```python
from build123d import *

# Parameters (mm, degrees)
SKETCH1_R           = 9
BOSS_EXTRUDE1_DEPTH = 66
SKETCH2_R           = 8.5
BOSS_EXTRUDE2_DEPTH = 2
SKETCH3_R           = 8
CUT_EXTRUDE1_DEPTH  = 1.5
SKETCH4_R           = 3
BOSS_EXTRUDE3_DEPTH = 1
FILLET1_R           = 1
CHAMFER1_SIZE       = 2


with BuildPart() as part:
    # Sketch1 → Boss-Extrude1 (new body)
    with BuildSketch(Plane.XY):
        Circle(SKETCH1_R)
    extrude(amount=BOSS_EXTRUDE1_DEPTH)

    # Sketch2 → Boss-Extrude2 (add)
    with BuildSketch(Plane(origin=(0, 0, 0), x_dir=(-1, 0, 0), z_dir=(0, 0, -1))):
        Circle(SKETCH2_R)
    extrude(amount=BOSS_EXTRUDE2_DEPTH)

    # Sketch3 → Cut-Extrude1 (cut)
    with BuildSketch(Plane(origin=(0, 0, -2), x_dir=(-1, 0, 0), z_dir=(0, 0, -1))):
        Circle(SKETCH3_R)
    extrude(amount=-CUT_EXTRUDE1_DEPTH, mode=Mode.SUBTRACT)

    # Sketch4 → Boss-Extrude3 (add)
    with BuildSketch(Plane(origin=(0, 0, -0.5), x_dir=(-1, 0, 0), z_dir=(0, 0, -1))):
        with Locations((0, 4)):
            Circle(SKETCH4_R)
        with Locations((0, -4)):
            Circle(SKETCH4_R)
    extrude(amount=BOSS_EXTRUDE3_DEPTH)

    # Fillet1
    fillet1_edges = [part.edges().sort_by_distance(p)[0] for p in [
        (3, 4, -1.5),
        (3, -4, -1.5),
    ]]
    fillet(fillet1_edges, radius=FILLET1_R - 0.0001)  # a hair under: the kernel refuses the full size

    # Chamfer1
    chamfer1_edges = [part.edges().sort_by_distance(p)[0] for p in [
        (-9, 0, 66),
    ]]
    chamfer(chamfer1_edges, length=CHAMFER1_SIZE)


solid = part.part
```
Design review of the part built by this model. Coordinates are the model's own, in mm. A direction names the side the tool comes from. Coordinates: 2 decimals unless noted, no trailing zeros. Loops run counter-clockwise (first coordinate to the right, second up) from the corner with the lowest first, then second, coordinate; pieces in that order, holes last. Notation, with made-up numbers: M 55,49 L 88,49 A13 cw 88,74 Z; hole C 76,-11.5 d1. An arc over 180 degrees is marked long. One line per question, with ' | ' between items.
(1) Wall thickness on probe 1 along Y at (x, z) = (0, -1.1); probe 2 along Y at (x, z) = (0, -1.2); probe 3 along Z at (x, y) = (2.5, 1.5): over which ranges is each line inside the solid? List them lowest first.
Filled in:
probe 1: y = -8.5 to -8, -6.8 to -1.2, 1.2 to 6.8, 8 to 8.5 | probe 2: y = -8.5 to -8, -6.71 to -1.29, 1.29 to 6.71, 8 to 8.5 | probe 3: z = -0.5 to 66
(2) Draft analysis for pull direction Y (two halves, no side actions). For faces 3 (the face through (-1.172, 8.923, 31.552)), 4 (the face through (0, -4, -1.5)), 5 (the face through (8, -3.3, 0)), state which applies: released by +Y, released by -Y, zero draft, split by the parting line, or undercut.
Filled in:
face 3: split by the parting line | face 4: undercut | face 5: zero draft
(3) We need section C-C (z = 37.5). Give the boundary of the cut face in (x, y), and give its area (3 significant figures).
Filled in:
outline: C 0,0 d18 | area: 254 mm^2
(4) For pin 1 Ø5 at (y, z) = (5.5, 37.5) entering from +X; pin 2 Ø8 at (x, y) = (-3, -1) entering from -Z; pin 3 Ø5 at (x, z) = (-7, 27) entering from +Y; pin 4 Ø8 at (y, z) = (-2.5, 39) entering from -X, all flat-tipped, find the tip position at first contact; note any pin that passes through.
Filled in:
pin 1: stops at x = 8.49 | pin 2: stops at z = -1.5 | pin 3: stops at y = 7.79 | pin 4: stops at x = -9
(5) Machinability: for faces 1 (the face through (0, 0, 66)), 2 (the face through (-4.57, 7.167, -0.986)), which of the approach directions +Z, -Z, +X, -X, +Y, -Y give a long, thin tool a straight path to every point of the face, cutting with its end or side? Answer none if there is none.
Filled in:
face 1: +Z, +X, -X, +Y, -Y | face 2: -Z
(6) We need section B-B (y = 0). Give the boundary of the cut face in (x, z), and give its area (3 significant figures).
Filled in:
outline: M -9,0 L -8.5,0 L -8.5,-2 L -8,-2 L -8,-0.5 L 8,-0.5 L 8,-2 L 8.5,-2 L 8.5,0 L 9,0 L 9,64 L 7,66 L -7,66 L -9,64 Z | area: 1,190 mm^2
